For this review, use the dimensioned drawing (mm, ordinates from the lowest corner) and the shaded views. Give positions to 0.01 mm unless a question says otherwise; leave off trailing zeros. Order: outer loops, then holes, each group sorted by start corner. A loop starts at its lowest first (then second) coordinate and runs counter-clockwise, first axis right, second up. Notation, with made-up numbers: (-37.75, -8.75) -> (-14.75, -8.75) arc R17 ccw to (-14.75, 9.25) -> close; hole circle Ø8 at (76.5, -3). An arc over 180 degrees is marked (long way). Return JSON: item names as keys, results as strings.
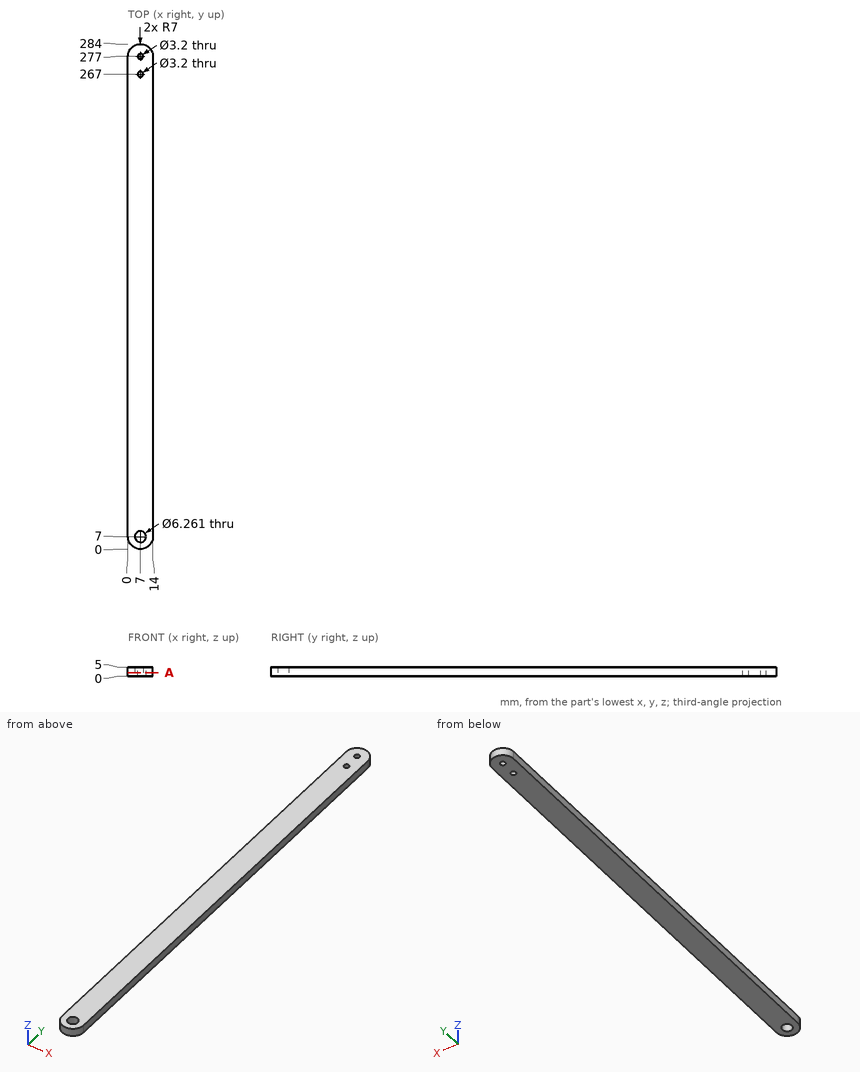
Item 1: Add section A-A (z = 1.95). Give the boundary of the cut face in (x, y), plus the area to 3 significant figures.
Result set:
{"outline": "(0, 7) arc R7 ccw to (14, 7) -> (14, 277) arc R7 ccw to (0, 277) -> close; hole circle Ø6.26 at (7, 7); hole circle Ø3.2 at (7, 267); hole circle Ø3.2 at (7, 277)", "area": "3,890 mm^2"}
Item 2: Wall thickness on L1, parallel to Y at x = 7, z = 1.3; L2, parallel to X at y = 277, z = 1.45; L3, parallel to Y at x = 8, z = 2.85: over which ranges is each line inside the solid? List them lowest first. Write a range as [from, to].
Result set:
{"L1": "y = [0, 3.87], [10.13, 265.4], [268.6, 275.4], [278.6, 284]", "L2": "x = [0, 5.4], [8.6, 14]", "L3": "y = [0.07, 4.03], [9.97, 265.75], [268.25, 275.75], [278.25, 283.93]"}
Item 3: For pin 1 (4 mm diameter, centred on x = 7, y = 7, fed in from +Z), flat-tipped, find the tip position at first contact; note if it passes through.
Result set:
{"pin 1": "passes through"}
